Design review of the part built by this model. Coordinates are the model's own, in mm. A direction names the side the tool comes from. Coordinates: 2 decimals unless noted, no trailing zeros. Loops run counter-clockwise (first coordinate to the right, second up) from the corner with the lowest first, then second, coordinate; pieces in that order, holes last. Notation, with made-up numbers: (21.5, 15) -> (32.5, 15) arc R10 cw to (32.5, 21) -> close; hole circle Ø11 at (19.25, 32.5). An arc over 180 degrees is marked (long way). Use a Markdown table: item, result. Add a question column.
Q1. For probe 1 along Y at (x, z) = (0, 13.5) (1 decimal); probe 2 along X at (y, z) = (-17, 14); probe 3 along Y at (x, z) = (-2.5, 5.25), list the stretches that pass through material, from the lowest coordinate up.
Q2. Take a section at A-A on y = 0. Write out the cut boundary in (x, z) (3 decimals).
Q3. Take a section at D-D on x = 0. Count the separate pieces of the cut face and the enclosed holes in it, plus the area to 3 significant figures.
Q4. Take a section at B-B on x = -13. Write out the cut boundary in (y, z).
Q5. For faces 1 (the face through (-0.46, -39.21, 8.75)), 2 (the face through (-1.595, 26.36, 10.133)), 3 (the face through (-3.556, 28, 13)), list the 3-axis set-ups (+Z, -Z, +X, -X, +Y, -Y) from which the entire face can be reached by the end or side of a thin tool; tool diameter is ignored.
Q6. Clearance check with flat-ended pins moving along their axes: pin 1 Ø3.5 at (y, z) = (-33.5, 11.5) entering from -X; pin 2 Ø0.9 at (x, y) = (0, 28.5) entering from +Z; pin 3 Ø10 at (y, z) = (-24.5, 9) entering from -X. State where each tip first meets the part, or that it passes through.
Q7. Draft analysis for pull direction Y (two halves, no side actions). For faces 4 (the face through (9.906, -35, 10)), 5 (the face through (2, -40.64, 9)), 6 (the face through (25.685, -16.299, 11.962)), state which applies: pulls with the +Y half, pulls with the -Y half, needs draft (parallel to the pull), parting line crosses it, or undercut.
Q8. Take a section at C-C on z = 17.25. Write out the cut boundary in (x, y) (1 decimal).
from build123d import *

# Parameters (mm, degrees)
SKETCH1_R                   = 30.988
BOSS_EXTRUDE1_DEPTH         = 19.05
SKETCH2_R                   = 26.035
CUT_EXTRUDE1_DEPTH          = 48.785089599
BOSS_EXTRUDE2_START         = -2.54
SKETCH4_R                   = 26.035
SKETCH4_R_2                 = 23.495
BOSS_EXTRUDE2_DEPTH         = 2.54
SKETCH11_W                  = 7.112
SKETCH11_H                  = 3.048
CUT_EXTRUDE3_DEPTH          = 11.938
CIRPATTERN2_COUNT           = 3
F_4_CLEARANCE_HOLE1_D       = 3.4544
F_4_CLEARANCE_HOLE1_DEPTH   = 34.456395212
SKETCH15_W                  = 19.05
SKETCH15_H                  = 17.653
BOSS_EXTRUDE3_DEPTH         = 12.7
CIRPATTERN3_COUNT           = 3
SKETCH16_W                  = 11.43
SKETCH16_H                  = 5.842
CUT_EXTRUDE4_DEPTH          = 55.322904735
CHAMFER2_SIZE               = 8.129699408
CHAMFER2_SIZE_2             = 5.08
F_1_4_CLEARANCE_HOLE1_D     = 7.14248
F_1_4_CLEARANCE_HOLE1_DEPTH = 2.811307748


with BuildPart() as part:
    # Sketch1 → Boss-Extrude1 (new body)
    with BuildSketch(Plane.XY):
        with Locations(Location((0, 0, 0), (0, 0, 180))):
            Circle(SKETCH1_R)
    extrude(amount=BOSS_EXTRUDE1_DEPTH)

    # Sketch2 → Cut-Extrude1 (cut, through all)
    with BuildSketch(Plane.XY.offset(19.05)):
        Circle(SKETCH2_R)
    extrude(amount=-CUT_EXTRUDE1_DEPTH, mode=Mode.SUBTRACT)

    # Sketch4 → Boss-Extrude2 (add)
    with BuildSketch(Plane(origin=(0, 0, 0), x_dir=(-1, 0, 0), z_dir=(0, 0, -1)).offset(BOSS_EXTRUDE2_START)):
        with Locations(Location((0, 0, 0), (0, 0, 180))):
            Circle(SKETCH4_R)
        Circle(SKETCH4_R_2, mode=Mode.SUBTRACT)
    extrude(amount=BOSS_EXTRUDE2_DEPTH)

    # Sketch11 → Cut-Extrude3 (cut)
    with BuildSketch(Plane.XY.offset(19.05)):
        with Locations((0, 28.2575)):
            Rectangle(SKETCH11_W, SKETCH11_H)
    cut_extrude3 = extrude(amount=-CUT_EXTRUDE3_DEPTH, mode=Mode.SUBTRACT)

    # CirPattern2: Cut-Extrude3 ×3 about axis
    cirpattern2_axis = Axis((0, 0, 0), (0, 0, 1))
    for i in range(1, CIRPATTERN2_COUNT):
        add(cut_extrude3.rotate(cirpattern2_axis, i * 360 / CIRPATTERN2_COUNT), mode=Mode.SUBTRACT)

    # #4 Clearance Hole1
    with Locations(Plane.XZ.offset(-12.7)):
        with Locations((0, 10.795)):
            f_4_clearance_hole1 = Hole(F_4_CLEARANCE_HOLE1_D / 2, depth=F_4_CLEARANCE_HOLE1_DEPTH)

    # Sketch15 → Boss-Extrude3 (add)
    with BuildSketch(Plane(origin=(0, -27.94, 0), x_dir=(1, 0, 0), z_dir=(0, 1, 0))):
        with Locations((0.381, -9.5885)):
            Rectangle(SKETCH15_W, SKETCH15_H)
    extrude(amount=-BOSS_EXTRUDE3_DEPTH)

    # CirPattern3: #4 Clearance Hole1 ×3 about axis
    cirpattern3_axis = Axis((0, 0, 19.05), (0, 0, 1))
    for i in range(1, CIRPATTERN3_COUNT):
        add(f_4_clearance_hole1.rotate(cirpattern3_axis, i * 360 / CIRPATTERN3_COUNT), mode=Mode.SUBTRACT)

    # Sketch16 → Cut-Extrude4 (cut, through all)
    with BuildSketch(Plane.XY.offset(18.415)):
        with Locations((0.381, -34.907692252)):
            Rectangle(SKETCH16_W, SKETCH16_H)
    extrude(amount=-CUT_EXTRUDE4_DEPTH, mode=Mode.SUBTRACT)

    # Chamfer2
    # the kernel refuses this chamfer: 8.129699408, 5.08 mm, written as the material it takes off along each edge
    with BuildSketch(Plane(origin=(-30.162101737, -40.64, 0.762), x_dir=(0, 0.9997899140358644, -0.020497019104217945), z_dir=(1, 0, 0))) as chamfer2_piece_1:
        Polygon((CHAMFER2_SIZE * 0.999789913978, CHAMFER2_SIZE * 0.020497019103), (-CHAMFER2_SIZE_2 * 0.0204970191042, CHAMFER2_SIZE_2 * 0.999789914036), (0, 0), align=None)
    extrude(amount=61.086203475, mode=Mode.SUBTRACT)

    # 1/4 Clearance Hole1
    with Locations(Plane(origin=(0, -40.64, 0), x_dir=(-1, 0, 0), z_dir=(0, -1, 0))):
        with Locations((0, -12.289529053)):
            Hole(F_1_4_CLEARANCE_HOLE1_D / 2, depth=F_1_4_CLEARANCE_HOLE1_DEPTH)


solid = part.part
Answer list:
| question | item | result |
|---|---|---|
| 1 | probe 1 | -32 to -26, 26 to 26.7, 29.8 to 31 |
| 1 | probe 2 | -25.91 to -24.57, -22.33 to -19.72, 19.72 to 22.33, 24.57 to 25.91 |
| 1 | probe 3 | -39.69 to -37.83, -31.99 to -25.91, 25.91 to 30.89 |
| 2 | outline | (-30.988, 0) -> (-23.495, 0) -> (-23.495, 2.54) -> (-26.035, 2.54) -> (-26.035, 19.05) -> (-30.988, 19.05) -> close; (23.495, 0) -> (30.988, 0) -> (30.988, 19.05) -> (26.035, 19.05) -> (26.035, 2.54) -> (23.495, 2.54) -> close |
| 3 | separate pieces | 6 |
| 3 | enclosed holes | 0 |
| 3 | area | 194 mm² |
| 4 | outline | (-28.13, 0) -> (-19.57, 0) -> (-19.57, 2.54) -> (-22.56, 2.54) -> (-22.56, 19.05) -> (-28.13, 19.05) -> close; (19.57, 0) -> (28.13, 0) -> (28.13, 19.05) -> (22.56, 19.05) -> (22.56, 2.54) -> (19.57, 2.54) -> close |
| 5 | face 1 | -Y |
| 5 | face 2 | +Y |
| 5 | face 3 | +Z |
| 6 | pin 1 | x = -9.14 |
| 6 | pin 2 | z = 7.11 |
| 6 | pin 3 | x = -24.08 |
| 7 | face 4 | needs draft |
| 7 | face 5 | pulls with the -Y half |
| 7 | face 6 | undercut |
| 8 | outline | (-9.1, -40.6) -> (9.9, -40.6) -> (9.9, -29.4) arc R31 ccw (long way) to (-9.1, -29.6) -> close; hole (-27.6, -11.8) -> (-24, -18) -> (-21.4, -16.4) -> (-24.9, -10.3) -> close; hole circle Ø52.1 at (0, 0); hole (-5.3, -37.8) -> (6.1, -37.8) -> (6.1, -32) -> (-5.3, -32) -> close; hole (-3.6, 26.7) -> (3.6, 26.7) -> (3.6, 29.8) -> (-3.6, 29.8) -> close; hole (21.4, -16.4) -> (24, -18) -> (27.6, -11.8) -> (24.9, -10.3) -> close |
